Geometry check sheet. Reference: the model listing, model coordinates, mm. A direction names the side the tool comes from. Round coordinates to 2 decimals unless told otherwise and drop trailing zeros. Order: outer loops, then holes, each group sorted by start corner. A loop starts at its lowest first (then second) coordinate and runs counter-clockwise, first axis right, second up. Notation, with made-up numbers: (16.5, 8.5) - (51.5, 8.5) arc R30 cw to (51.5, 38.5) - close; hole circle Ø9 at (-22, -0.75). An arc over 180 degrees is marked (long way). Answer as CSV lines item,"result". Start each with the question number.
Autodesk Inventor part; units mm, degrees
ref_plane "YZ Plane" through (0, 0, 0) normal (1, 0, 0) x (0, 1, 0)
ref_plane "XZ Plane" through (0, 0, 0) normal (0, 1, 0) x (-1, 0, 0)
ref_plane "XY Plane" through (0, 0, 0) normal (0, 0, 1) x (1, 0, 0)
sketch "Sketch1" plane through (0, 0, 0) normal (0, 0, 1) x (1, 0, 0)
  line L0 (14, 12.3) -> (14, 0)
  line L1 (14, 0) -> (0, 0)
  line L2 (0, 0) -> (0, 6.3)
  line L3 (-5.5, 12.3) -> (14, 12.3)
  line L4 (0, 6.3) -> (-5.5, 6.3)
  line L5 (-5.5, 6.3) -> (-5.5, 12.3)
  dimension "d1" = 6.3
  dimension "d2" = 6
  dimension "d4" = 14
  dimension "d5" = 5.5
extrude "Extrusion1" add sketch "Sketch1" along normal blind 280
sketch "Sketch2" plane through (-5.5, 12.3, 0) normal (0, 1, 0) x (1, 0, 0)
  circle A0 centre (12.5, -270) radius 2.5
  circle A1 centre (12.5, -10) radius 2.5
  circle A2 centre (12.5, -190) radius 2.5
  line L0 (19.5, -280) -> (0, -280)
  line L1 (19.5, 0) -> (19.5, -280)
  line L2 (19.5, 0) -> (0, 0)
  circle A3 centre (12.5, -90) radius 2.5
  point P0 (5.5, 0)
  dimension "d8" = 5
  dimension "d9" = 10
  dimension "d10" = 7
  dimension "d11" = 10
  dimension "d12" = 7
  dimension "d13" = 7
  dimension "d14" = 90
  dimension "d15" = 5
  dimension "d16" = 90
  dimension "d17" = 7
extrude "Extrusion2" cut sketch "Sketch2" against normal through all
fillet "Fillet1" radius 1 1 edges at (0, 6.3, 140)
properties part number "1324_Clamp Rail_V1" material "Acetal Resin, White"
1. Section check B-B on y = 3.25. Record the boundary of the cut face in (x, z).
2. Section check C-C on x = 7. Record the boundary of the cut face in (y, z), plus the area to 3 significant figures.
3. Thickness scan on probe 1 along Z at (x, y) = (7, 8.5); probe 2 along X at (y, z) = (7.5, 90); probe 3 along Z at (x, y) = (7.75, 11.75). Record the ranges inside material, lowest first.
4. Section check D-D on z = 223. Record the boundary of the cut face in (x, y), plus the area to 3 significant figures.
5. Go/stop test with flat-tipped pins: pin 1 Ø3 at (y, z) = (3.5, 172.5) entering from -X; pin 2 Ø2 at (x, z) = (-2.5, 81.5) entering from -Y. Record where each tip stops, or that it passes through.
6. Draft check along Z on faces 1 (the face through (8.15, 6.24, 12.22)), 2 (the face through (-3, 6.3, 138)), 3 (the face through (6, 6, 0)). Enter one of: released by +Z, released by -Z, zero draft, split by the parting line, or undercut.
7. Section check A-A on z = 270. Record the boundary of the cut face in (x, y).
8. Access from +Z, -Z, +X, -X, +Y, -Y to the whole of each face (thin tool, end or side, straight path). Record for faces 4 (the face through (14, 6, 138)), 5 (the face through (0, 3, 138)).
Numbers:
1,outline,"(0, 0) - (14, 0) - (14, 280) - (0, 280) - close; hole circle Ø5 at (7, 10); hole circle Ø5 at (7, 90); hole circle Ø5 at (7, 190); hole circle Ø5 at (7, 270)"
2,outline,"(0, 0) - (12.3, 0) - (12.3, 7.5) - (0, 7.5) - close; (0, 12.5) - (12.3, 12.5) - (12.3, 87.5) - (0, 87.5) - close; (0, 92.5) - (12.3, 92.5) - (12.3, 187.5) - (0, 187.5) - close; (0, 192.5) - (12.3, 192.5) - (12.3, 267.5) - (0, 267.5) - close; (0, 272.5) - (12.3, 272.5) - (12.3, 280) - (0, 280) - close"
2,area,"3,200 mm2"
3,probe 1,"z = 0 to 7.5, 12.5 to 87.5, 92.5 to 187.5, 192.5 to 267.5, 272.5 to 280"
3,probe 2,"x = -5.5 to 4.5, 9.5 to 14"
3,probe 3,"z = 0 to 7.62, 12.38 to 87.62, 92.38 to 187.62, 192.38 to 267.62, 272.38 to 280"
4,outline,"(-5.5, 6.3) - (-1, 6.3) arc R1 cw to (0, 5.3) - (0, 0) - (14, 0) - (14, 12.3) - (-5.5, 12.3) - close"
4,area,"205 mm2"
5,pin 1,"stops at x = 0"
5,pin 2,"stops at y = 6.3"
6,face 1,"undercut"
6,face 2,"zero draft"
6,face 3,"released by -Z"
7,outline,"(-5.5, 6.3) - (-1, 6.3) arc R1 cw to (0, 5.3) - (0, 0) - (4.5, 0) - (4.5, 12.3) - (-5.5, 12.3) - close; (9.5, 0) - (14, 0) - (14, 12.3) - (9.5, 12.3) - close"
8,face 4,"+Z, -Z, +X, +Y, -Y"
8,face 5,"+Z, -Z, -X, -Y"
